from build123d import *

# Parameters (mm, degrees)
F1_DEPTH       = 28.575
F3_D           = 5.5626
F3_DEPTH       = 11.43
F3_CBORE_D     = 6.858
F3_CBORE_DEPTH = 5.08
F3_TIP         = 1.6711736397


with BuildPart() as f1:
    # F0 (on Top) → F1 (new body)
    with BuildSketch(Plane.XY):
        with BuildLine():
            Line((2.4528223929, 7.5490110981), (0.9736080693, 9.3150838242))
            ThreePointArc((0.9736080693, 9.3150838242), (0, 9.7696162728), (-0.9736080693, 9.3150838242))
            Line((-0.9736080693, 9.3150838242), (-2.4528223929, 7.5490110981))
            Line((-2.4528223929, 7.5490110981), (-4.6876034218, 8.1083335825))
            ThreePointArc((-4.6876034218, 8.1083335825), (-5.7424363657, 7.9037855932), (-6.2629343697, 6.9637886532))
            Line((-6.2629343697, 6.9637886532), (-6.4215723929, 4.6655454401))
            Line((-6.4215723929, 4.6655454401), (-8.5583097316, 3.8044755043))
            ThreePointArc((-8.5583097316, 3.8044755043), (-9.291457218, 3.0189774568), (-9.1600326102, 1.9525629071))
            Line((-9.1600326102, 1.9525629071), (-7.9375, 0))
            Line((-7.9375, 0), (-9.1600326102, -1.9525629071))
            ThreePointArc((-9.1600326102, -1.9525629071), (-9.291457218, -3.0189774568), (-8.5583097316, -3.8044755043))
            Line((-8.5583097316, -3.8044755043), (-6.4215723929, -4.6655454401))
            Line((-6.4215723929, -4.6655454401), (-6.2629343697, -6.9637886532))
            ThreePointArc((-6.2629343697, -6.9637886532), (-5.7424363657, -7.9037855932), (-4.6876034218, -8.1083335825))
            Line((-4.6876034218, -8.1083335825), (-2.4528223929, -7.5490110981))
            Line((-2.4528223929, -7.5490110981), (-0.9736080693, -9.3150838242))
            ThreePointArc((-0.9736080693, -9.3150838242), (0, -9.7696162728), (0.9736080693, -9.3150838242))
            Line((0.9736080693, -9.3150838242), (2.4528223929, -7.5490110981))
            Line((2.4528223929, -7.5490110981), (4.6876034218, -8.1083335825))
            ThreePointArc((4.6876034218, -8.1083335825), (5.7424363657, -7.9037855932), (6.2629343697, -6.9637886532))
            Line((6.2629343697, -6.9637886532), (6.4215723929, -4.6655454401))
            Line((6.4215723929, -4.6655454401), (8.5583097316, -3.8044755043))
            ThreePointArc((8.5583097316, -3.8044755043), (9.291457218, -3.0189774568), (9.1600326102, -1.9525629071))
            Line((9.1600326102, -1.9525629071), (7.9375, 0))
            Line((7.9375, 0), (9.1600326102, 1.9525629071))
            ThreePointArc((9.1600326102, 1.9525629071), (9.291457218, 3.0189774568), (8.5583097316, 3.8044755043))
            Line((8.5583097316, 3.8044755043), (6.4215723929, 4.6655454401))
            Line((6.4215723929, 4.6655454401), (6.2629343697, 6.9637886532))
            ThreePointArc((6.2629343697, 6.9637886532), (5.7424363657, 7.9037855932), (4.6876034218, 8.1083335825))
            Line((4.6876034218, 8.1083335825), (2.4528223929, 7.5490110981))
        make_face()
    extrude(amount=F1_DEPTH)

    # F3
    with Locations(Plane(origin=(0, 0, 0), x_dir=(1, 0, 0), z_dir=(0, 0, -1))):
        with Locations((0, 0)):
            CounterBoreHole(F3_D / 2, F3_CBORE_D / 2, F3_CBORE_DEPTH, depth=F3_DEPTH)
            with Locations((0, 0, -(F3_DEPTH + F3_TIP / 2))):  # 118° drill point
                Cone(0, F3_D / 2, F3_TIP, mode=Mode.SUBTRACT)


solid = f1.part
Geometry check sheet. Reference: the model listing, model coordinates, mm. A direction names the side the tool comes from. Round coordinates to 2 decimals unless told otherwise and drop trailing zeros. Write each loop counter-clockwise with the first axis right and the second up, starting at its lowest first coordinate (ties: lowest second). Pieces come first, ordered by that corner, then holes. Notation, with made-up numbers: (31, 73) - (84, 73) arc R16 cw to (84, 80) - close; hole circle Ø6 at (-4.5, -10). An arc over 180 degrees is marked (long way). One line per item, written item: value.
1. Mould release check, pull along Y, two halves, no side actions. Record for faces 1 (the face through (0, 0, 28.575)), 2 (the face through (7.475, -4.241, 14.087)), 3 (the face through (-8.54, -0.96, 14.09)), 4 (the face through (5.755, 7.895, 14.087)): released by +Y, released by -Y, zero draft, split by the parting line, or undercut.
The answers:
face 1: zero draft
face 2: released by -Y
face 3: undercut
face 4: released by +Y
2. Depth check by flat-ended pin: pin 1 Ø1.5 at (y, z) = (7.5, 16.5) entering from -X; pin 2 Ø3 at (x, z) = (-4.5, 13) entering from +Y. Enter the tip coordinate at first touch or a pass-through.
The answers:
pin 1: stops at x = -6.28
pin 2: stops at y = 8.15
3. Set-up check for faces 5 (the face through (6.343, 5.799, 14.087)), 6 (the face through (-1.703, 8.444, 14.087)), 7 (the face through (-7.5, -4.23, 14.09)), 8 (the face through (0, -3, 5.08)), 9 (the face through (8.557, -0.99, 14.087)): record each of +Z, -Z, +X, -X, +Y, -Y from which the full face is reachable in a straight line by a thin tool's end or side.
The answers:
face 5: +Z, -Z, +X, +Y
face 6: +Z, -Z, +Y
face 7: +Z, -Z, -X, -Y
face 8: -Z
face 9: +Z, -Z, +X
4. Scan lines: L1, parallel to Y at x = 0, z = 1.9; L2, parallel to Y at x = 0, z = 9.75; L3, parallel to Y at x = 5, z = 15.75. Record each from-to range of solid material in increasing order.
The answers:
L1: y = -9.77 to -3.43, 3.43 to 9.77
L2: y = -9.77 to -2.78, 2.78 to 9.77
L3: y = -8.15 to 8.15
5. Cross-section at D-D on x = -7. Record the boundary of the cut face in (y, z) (3 decimals), and give its area (3 significant figures).
The answers:
outline: (-4.432, 0) - (4.432, 0) - (4.432, 28.575) - (-4.432, 28.575) - close
area: 253 mm^2
